The model under review builds one solid part; all positions refer to its coordinate system, in mm. Face numbers are marked on the shaded views. Coordinates: 2 decimals unless noted, no trailing zeros. Loops run counter-clockwise (first coordinate to the right, second up) from the corner with the lowest first, then second, coordinate; pieces in that order, holes last. Notation, with made-up numbers: (12, 44) - (38, 44) arc R13 cw to (38, 54) - close; hole circle Ø4 at (-28, 77). An arc over 180 degrees is marked (long way). Use a Markdown table: item, result. Add a question column.
1) Clearance check with flat-ended pins moving along their axes: pin 1 (4.5 mm diameter, centred on x = 63.75, y = 8.25, fed in from -Z); pin 2 (8 mm diameter, centred on x = 31, y = 5, fed in from -Z); pin 3 (3 mm diameter, centred on x = -9, y = 7, fed in from -Z); pin 4 (5.5 mm diameter, centred on y = -12, z = 1.5, fed in from -X). State where each tip first meets the part, or that it passes through.
2) Add section A-A, the plane x = -63.75. Give the boundary of the cut face in (y, z), and give its area (4 significant figures).
3) Add section D-D, the plane x = 55.5. Give the boundary of the cut face in (y, z), and give its area (4 significant figures).
4) Add section C-C, the plane y = -7. Give the boundary of the cut face in (x, z).
5) The part is to be moulded in two halves that separate along Z. For the marked faces 1 and 2, say which applies: pulls with the +Z half, pulls with the -Z half, needs draft (parallel to the pull), parting line crosses it, or undercut.
6) To check wall thickness, follow L1, parallel to X at y = -12, z = 1.75; L2, parallel to Y at x = 7, z = 4.05; L3, parallel to Y at x = -49.75, z = 2.3. State the ranges of each line that lie inside material, in increasing order. Write a range as [from, to].
7) Add section B-B, the plane z = 1.5. Give the boundary of the cut face in (x, y).
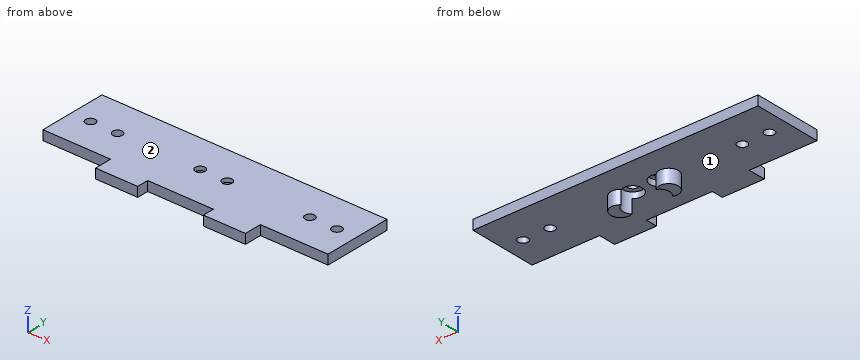
```python
from build123d import *

# Parameters (mm, degrees)
SKETCH1_W           = 147.5
SKETCH1_H           = 53.5
BOSS_EXTRUDE1_DEPTH = 5
SKETCH2_R           = 5
BOSS_EXTRUDE2_DEPTH = 7
SKETCH3_W           = 35
SKETCH3_H           = 18
CUT_EXTRUDE1_DEPTH  = 80.363877173
SKETCH4_W           = 34
SKETCH4_H           = 15
CUT_EXTRUDE2_DEPTH  = 10
SKETCH5_R           = 2.5
CUT_EXTRUDE3_DEPTH  = 80.363877173
SKETCH6_R           = 5
CUT_EXTRUDE4_DEPTH  = 10
SKETCH7_W           = 77.5
SKETCH7_H           = 9
CUT_EXTRUDE5_DEPTH  = 10


with BuildPart() as part:
    # Sketch1 → Boss-Extrude1 (new body)
    with BuildSketch(Plane.XY):
        Rectangle(SKETCH1_W, SKETCH1_H)
    extrude(amount=BOSS_EXTRUDE1_DEPTH)

    # Sketch2 → Boss-Extrude2 (add)
    with BuildSketch(Plane(origin=(0, 0, 0), x_dir=(-1, 0, 0), z_dir=(0, 0, -1))):
        with Locations(Location((12.5, 9.25, 0), (0, 0, 180))):
            Circle(SKETCH2_R)
        with Locations(Location((-12.5, 9.25, 0), (0, 0, 180))):
            Circle(SKETCH2_R)
    extrude(amount=BOSS_EXTRUDE2_DEPTH)

    # Sketch3 → Cut-Extrude1 (cut, through all)
    with BuildSketch(Plane.XY.offset(5)):
        with Locations((-56.25, -17.75)):
            Rectangle(SKETCH3_W, SKETCH3_H)
        with Locations((56.25, -17.75)):
            Rectangle(SKETCH3_W, SKETCH3_H)
    extrude(amount=-CUT_EXTRUDE1_DEPTH, mode=Mode.SUBTRACT)

    # Sketch4 → Cut-Extrude2 (cut)
    with BuildSketch(Plane.XY.offset(5)):
        with Locations((0, -19.25)):
            Rectangle(SKETCH4_W, SKETCH4_H)
    extrude(amount=-CUT_EXTRUDE2_DEPTH, mode=Mode.SUBTRACT)

    # Sketch5 → Cut-Extrude3 (cut, through all)
    with BuildSketch(Plane.XY.offset(5)):
        with Locations((63.75, 8.25)):
            Circle(SKETCH5_R)
        with Locations((49.75, 8.25)):
            Circle(SKETCH5_R)
        with Locations((7, 8.25)):
            Circle(SKETCH5_R)
        with Locations((-49.75, 8.25)):
            Circle(SKETCH5_R)
        with Locations((-63.75, 8.25)):
            Circle(SKETCH5_R)
        with Locations((-7, 8.25)):
            Circle(SKETCH5_R)
    extrude(amount=-CUT_EXTRUDE3_DEPTH, mode=Mode.SUBTRACT)

    # Sketch6 → Cut-Extrude4 (cut)
    with BuildSketch(Plane(origin=(0, 0, -7), x_dir=(-1, 0, 0), z_dir=(0, 0, -1))):
        with Locations((7, 8.25)):
            Circle(SKETCH6_R)
        with Locations((-7, 8.25)):
            Circle(SKETCH6_R)
    extrude(amount=-CUT_EXTRUDE4_DEPTH, mode=Mode.SUBTRACT)

    # Sketch7 → Cut-Extrude5 (cut)
    with BuildSketch(Plane.XY.offset(5)):
        with Locations((0, -22.25)):
            Rectangle(SKETCH7_W, SKETCH7_H)
    extrude(amount=-CUT_EXTRUDE5_DEPTH, mode=Mode.SUBTRACT)


solid = part.part
```
From the geometry:
| question | item | result |
|---|---|---|
| 1 | pin 1 | passes through |
| 1 | pin 2 | stops at z = 0 |
| 1 | pin 3 | stops at z = 3 |
| 1 | pin 4 | stops at x = -38.75 |
| 2 | outline | (-8.75, 0) - (5.75, 0) - (5.75, 5) - (-8.75, 5) - close; (10.75, 0) - (26.75, 0) - (26.75, 5) - (10.75, 5) - close |
| 2 | area | 152.5 mm^2 |
| 3 | outline | (-8.75, 0) - (26.75, 0) - (26.75, 5) - (-8.75, 5) - close |
| 3 | area | 177.5 mm^2 |
| 4 | outline | (-73.75, 0) - (73.75, 0) - (73.75, 5) - (-73.75, 5) - close |
| 5 | face 1 | pulls with the -Z half |
| 5 | face 2 | pulls with the +Z half |
| 6 | L1 | x = [-38.75, -17], [17, 38.75] |
| 6 | L2 | y = [-11.75, 5.75], [10.75, 26.75] |
| 6 | L3 | y = [-8.75, 5.75], [10.75, 26.75] |
| 7 | outline | (-73.75, -8.75) - (-38.75, -8.75) - (-38.75, -17.75) - (-17, -17.75) - (-17, -11.75) - (17, -11.75) - (17, -17.75) - (38.75, -17.75) - (38.75, -8.75) - (73.75, -8.75) - (73.75, 26.75) - (-73.75, 26.75) - close; hole circle Ø5 at (-63.75, 8.25); hole circle Ø5 at (-49.75, 8.25); hole circle Ø10 at (-7, 8.25); hole circle Ø10 at (7, 8.25); hole circle Ø5 at (49.75, 8.25); hole circle Ø5 at (63.75, 8.25) |
